For this review, use the dimensioned drawing (mm, ordinates from the lowest corner) and the shaded views. Coordinates: 2 decimals unless noted, no trailing zeros. Loops run counter-clockwise (first coordinate to the right, second up) from the corner with the lowest first, then second, coordinate; pieces in that order, holes last. Notation, with made-up numbers: (53.25, 25) -> (76.25, 25) arc R29 ccw to (76.25, 57) -> close; hole circle Ø9 at (78.5, 10.25). An arc over 180 degrees is marked (long way). Answer as a JSON object with one key per item and string values.
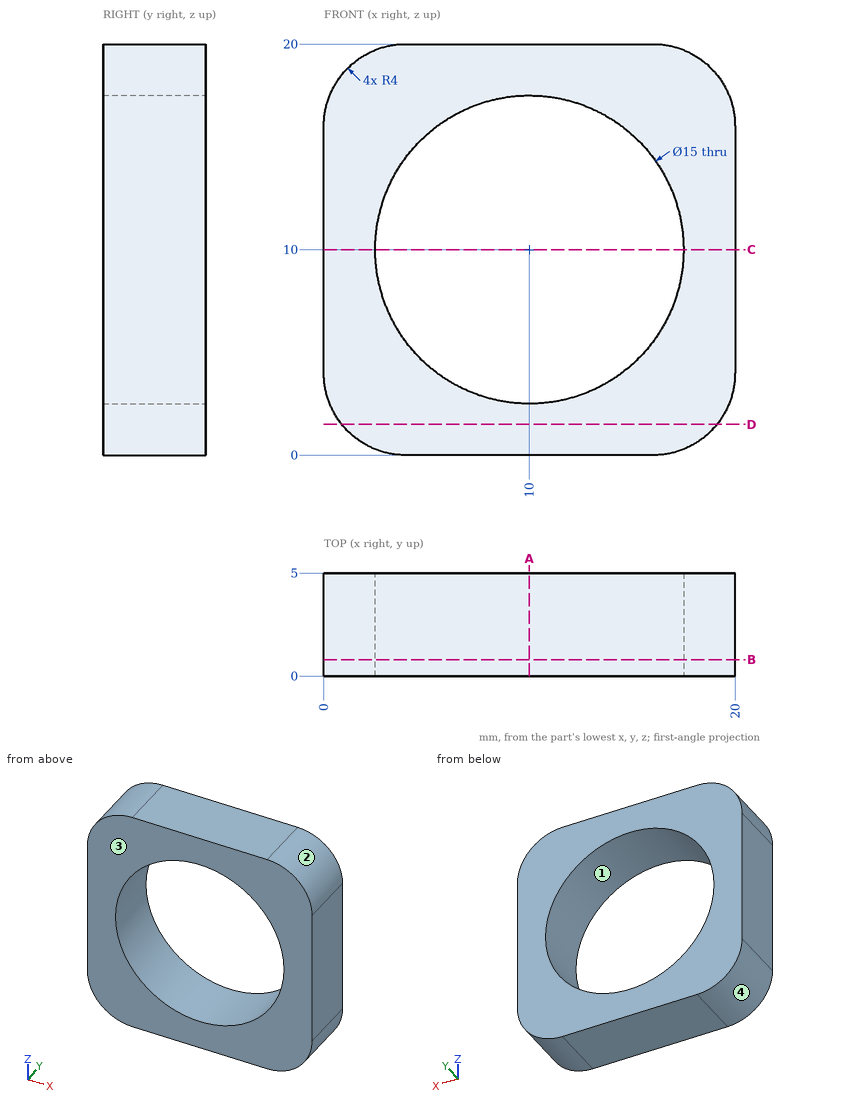
1) Add section D-D, the plane z = 1.5. Give the boundary of the cut face in (x, y).
Completed:
{"outline": "(0.88, 0) -> (19.12, 0) -> (19.12, 5) -> (0.88, 5) -> close"}
2) Clearance check with a flat-ended pin moving along its axis: pin 1 Ø1 at (x, z) = (5, 11) entering from -Y. State where the tip first meets the part, or that it passes through.
Completed:
{"pin 1": "through"}
3) Add section A-A, the plane x = 10. Give the boundary of the cut face in (y, z), and give its area (3 significant figures).
Completed:
{"outline": "(0, 0) -> (5, 0) -> (5, 2.5) -> (0, 2.5) -> close; (0, 17.5) -> (5, 17.5) -> (5, 20) -> (0, 20) -> close", "area": "25.0 mm²"}
4) Add section B-B, the plane y = 0.8. Give the boundary of the cut face in (x, z).
Completed:
{"outline": "(0, 4) arc R4 ccw to (4, 0) -> (16, 0) arc R4 ccw to (20, 4) -> (20, 16) arc R4 ccw to (16, 20) -> (4, 20) arc R4 ccw to (0, 16) -> close; hole circle Ø15 at (10, 10)"}
5) The part is to be moulded in two halves that separate along X. For the marked faces 1, 2, 3 and 4, say which applies: pulls with the +X half, pulls with the -X half, needs draft (parallel to the pull), parting line crosses it, or undercut.
Completed:
{"face 1": "undercut", "face 2": "pulls with the +X half", "face 3": "needs draft", "face 4": "pulls with the -X half"}
6) Add section C-C, the plane z = 10. Give the boundary of the cut face in (x, y).
Completed:
{"outline": "(0, 0) -> (2.5, 0) -> (2.5, 5) -> (0, 5) -> close; (17.5, 0) -> (20, 0) -> (20, 5) -> (17.5, 5) -> close"}
7) Wall thickness on probe 1 along Z at (x, y) = (10, 1.6); probe 2 along Z at (x, y) = (8, 2.15): over which ranges is each line inside the solid? List them lowest first.
Completed:
{"probe 1": "0 to 2.5, 17.5 to 20", "probe 2": "0 to 2.77, 17.23 to 20"}
